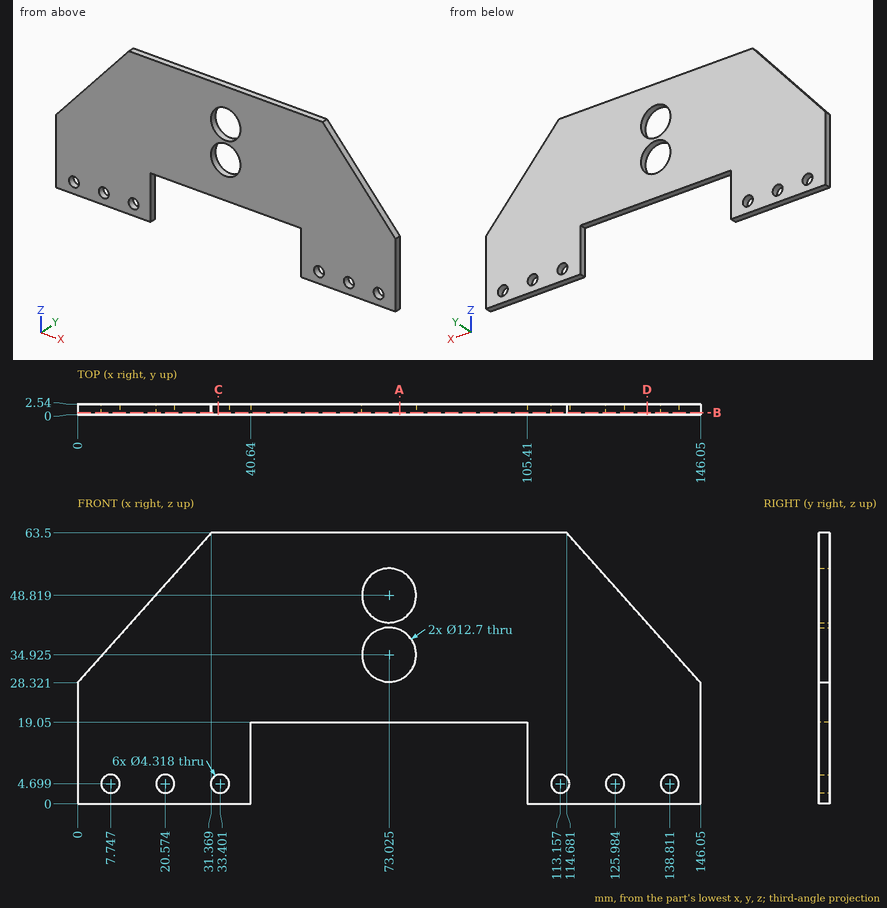
Can you work these out from the drawing? Everything is in mm from the part's minimum corner. Round coordinates to 2 decimals unless told otherwise and drop trailing zeros. Loops run counter-clockwise (first coordinate to the right, second up) from the corner with the lowest first, then second, coordinate; pieces in that order, holes last. Notation, with made-up numbers: M 1,29 L 39,29 A17 ccw 39,54 Z; hole C -33.5,6.25 d1. An arc over 180 degrees is marked long. Answer in a Markdown table with one row per item.
1. If we section it at B-B, the plane y = 0.5: Give the number of separate pieces and of enclosed holes in the cut face, plus the area to 3 significant figures.
Established:
| item | result |
|---|---|
| separate pieces | 1 |
| enclosed holes | 8 |
| area | 6,600 mm² |
2. I'm going to push flat-ended pins straight in: pin 1 Ø1.5 at (y, z) = (2.5, 45) entering from -X; pin 2 Ø0.8 at (x, y) = (84, 1) entering from -Z. Where does each tip first touch, or does it pass through?
Established:
| item | result |
|---|---|
| pin 1 | x = 14.2 |
| pin 2 | z = 19.05 |
3. If we section it at A-A, the plane x = 75.5: Please give me the cut outline in (y, z), plus the area to 3 significant figures.
Established:
| item | result |
|---|---|
| outline | M 0,19.05 L 2.54,19.05 L 2.54,29.08 L 0,29.08 Z; M 0,40.77 L 2.54,40.77 L 2.54,42.97 L 0,42.97 Z; M 0,54.67 L 2.54,54.67 L 2.54,63.5 L 0,63.5 Z |
| area | 53.5 mm² |
4. If we section it at C-C, the plane x = 33: Please give me the cut outline in (y, z).
Established:
| item | result |
|---|---|
| outline | M 0,0 L 2.54,0 L 2.54,2.58 L 0,2.58 Z; M 0,6.82 L 2.54,6.82 L 2.54,63.5 L 0,63.5 Z |
5. If we section it at D-D, the plane x = 133.5: Please give me the cut outline in (y, z) (1 decimal).
Established:
| item | result |
|---|---|
| outline | M 0,0 L 2.5,0 L 2.5,42.4 L 0,42.4 Z |
6. Please list where these lines run through material, in increasing order: line 1 (X direction, y = 1.65, z = 8); line 2 (Z direction, x = 86.5, y = 1); line 3 (X direction, y = 0.7, z = 51). Write a range as from..to.
Established:
| item | result |
|---|---|
| line 1 | 0..40.64, 105.41..146.05 |
| line 2 | 19.05..63.5 |
| line 3 | 20.22..67.06, 78.99..125.83 |
